Check sheet for the modelled part. Datum: model origin and axes. Units: mm. Face numbers are marked on the shaded views. A direction names the side the tool comes from. Coordinates: 2 decimals unless noted, no trailing zeros. Loops run counter-clockwise (first coordinate to the right, second up) from the corner with the lowest first, then second, coordinate; pieces in that order, holes last. Notation, with made-up numbers: (3.5, 10.25) - (46.5, 10.25) arc R29 ccw to (46.5, 33.25) - close; hole circle Ø2 at (89.25, 16.25). An arc over 180 degrees is marked (long way). Write each question's results on one line, items separated by ' | '. Start each with the question number.
1. Cross-section at C-C (z = -91.5). Record the cut outline in (x, y).
2. Tool access check on the marked faces 1 and 2. Record the directions out of +Z, -Z, +X, -X, +Y, -Y that give a thin tool (end or side, any length) a straight path to the whole face; none if there is none.
3. Thickness scan on line 1 (Y direction, x = -44, z = -1); line 2 (Z direction, x = -59, y = 76.5); line 3 (Y direction, x = -13, z = -303). Record the ranges inside material, lowest first. Write a range as [from, to].
4. Gauge pin test, flat ends, axial feed: P1, Ø8, axis at x = -248, z = -199, coming from the +Y side; P2, Ø7, axis at x = -13.3, y = 179.98, coming from the +Z side; P3, Ø1, axis at y = 183.5, z = -0.5, coming from the -X side. Record the tip position at first contact, or that the pin passes through.
5. Cross-section at B-B (x = -179). Record the cut outline in (y, z).
6. Cross-section at D-D (y = 57). Record the cut outline in (x, z).
7. Cross-section at A-A (y = 98). Record the cut outline in (x, z).
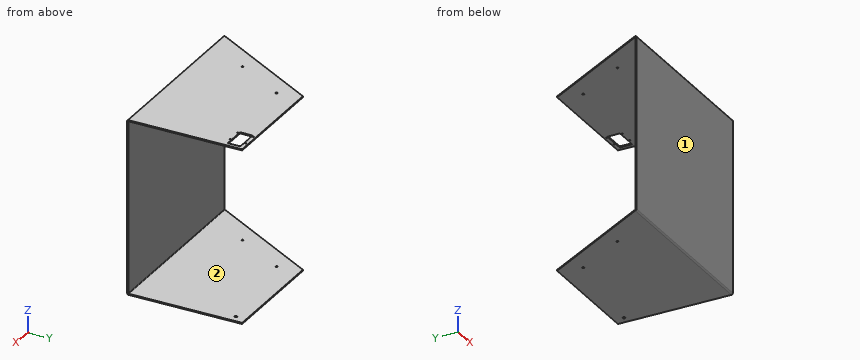
```python
from build123d import *

# Parameters (mm, degrees)
BASE_FLANGE2_DEPTH           = 2
EDGE_FLANGE1_DEPTH           = 309.908043232
EDGE_FLANGE2_STRIP_W         = 9
EDGE_FLANGE2_STRIP_H         = 2
EDGE_FLANGE2_STRIP_CUT_DEPTH = 309.908043232
EDGE_FLANGE2_DEPTH           = 309.908043232
SKETCH23_OUTSIDE_W           = 414.366
SKETCH23_OUTSIDE_H           = 376.458
CUT_EXTRUDE3_DEPTH           = 510.781566222
M3_CLEARANCE_HOLE1_REACH     = 479.133
M3_CLEARANCE_HOLE1_BORE_R    = 1.7
SKETCH50_R                   = 1.2
SKETCH50_W                   = 40
SKETCH50_H                   = 22
CUT_EXTRUDE5_DEPTH           = 10
FILLET1_R                    = 1.5
M4_CLEARANCE_HOLE2_D         = 4.3
M3_CLEARANCE_HOLE2_REACH     = 479.133
M3_CLEARANCE_HOLE2_BORE_R    = 1.7


# Sheet-metal steps are written as plain solids
with BuildPart() as part:
    # Sketch7 → Base-Flange2 (new body)
    with BuildSketch(Plane.XY):
        Polygon((-309.908043232, 0), (-195.602983964, 197.982170213), (0, 197.982170213), (0, 0), align=None)
    extrude(amount=-BASE_FLANGE2_DEPTH)

    # Edge-Flange1 section (across the edge) → Edge-Flange1 (add)
    with BuildSketch(Plane(origin=(0, -0.5, -2), x_dir=(0, 1, 0), z_dir=(-1, 0, 0))):
        with BuildLine():
            Line((-2, 0.5), (-2, 300))
            Line((-2, 300), (0, 300))
            Line((0, 300), (0, 0.5))
            ThreePointArc((0, 0.5), (0.146446609, 0.146446609), (0.5, 0))
            Line((0.5, 0), (0.5, -2))
            ThreePointArc((0.5, -2), (-1.267766953, -1.267766953), (-2, 0.5))
        make_face()
    extrude(amount=EDGE_FLANGE1_DEPTH)

    # Edge-Flange2 strip (across the edge) → Edge-Flange2 strip cut (cut)
    with BuildSketch(Plane(origin=(0, -0.5, -302), x_dir=(0, 0, 1), z_dir=(-1, 0, 0))):
        with Locations((-4, -1)):
            Rectangle(EDGE_FLANGE2_STRIP_W, EDGE_FLANGE2_STRIP_H)
    extrude(amount=EDGE_FLANGE2_STRIP_CUT_DEPTH, mode=Mode.SUBTRACT)

    # Edge-Flange2 section (across the edge) → Edge-Flange2 (add)
    with BuildSketch(Plane(origin=(0, -0.5, -302), x_dir=(0, 0, 1), z_dir=(-1, 0, 0))):
        with BuildLine():
            Line((-2, 0.5), (-2, 270))
            Line((-2, 270), (0, 270))
            Line((0, 270), (0, 0.5))
            ThreePointArc((0, 0.5), (0.146446609, 0.146446609), (0.5, 0))
            Line((0.5, 0), (0.5, -2))
            ThreePointArc((0.5, -2), (-1.267766953, -1.267766953), (-2, 0.5))
        make_face()
    extrude(amount=EDGE_FLANGE2_DEPTH)

    # Sketch23 outside → Cut-Extrude3 (cut, through all)
    with BuildSketch(Plane.XY.offset(-302)):
        with Locations((-154.954, 133.5)):
            Rectangle(SKETCH23_OUTSIDE_W, SKETCH23_OUTSIDE_H)
        Polygon((-309.908043232, 0), (-195.602983964, 197.982170213), (0, 197.982170213), (0, 0), (15.914954138, -38.535343566), (-328.412515317, -22.782185248), align=None, mode=Mode.SUBTRACT)
    extrude(amount=-CUT_EXTRUDE3_DEPTH, mode=Mode.SUBTRACT)

    # M3 Clearance Hole1 bore → M3 Clearance Hole1 (cut, up to next)
    with BuildSketch(Plane(origin=(0, 0, -304), x_dir=(-1, 0, 0), z_dir=(0, 0, -1)), mode=Mode.PRIVATE) as m3_clearance_hole1_sk1:
        with Locations((235.596855298, 71.137815764)):
            Circle(M3_CLEARANCE_HOLE1_BORE_R)
    m3_clearance_hole1_tool1 = extrude(m3_clearance_hole1_sk1.sketch, amount=-M3_CLEARANCE_HOLE1_REACH, mode=Mode.PRIVATE) & part.part
    m3_clearance_hole1 = m3_clearance_hole1_tool1.solids().sort_by_distance((-235.596855, 71.137816, -304))[0]
    add(m3_clearance_hole1, mode=Mode.SUBTRACT)

    # Mirror3: M3 Clearance Hole1 across plane
    add(m3_clearance_hole1.mirror(Plane.XY.offset(-152)), mode=Mode.SUBTRACT)

    # Sketch50 → Cut-Extrude5 (cut)
    with BuildSketch(Plane.XY):
        with Locations((-20, 193.482170213)):
            Circle(SKETCH50_R)
        with Locations((-20, 166.482170213)):
            Circle(SKETCH50_R)
        with Locations((-44, 193.482170213)):
            Circle(SKETCH50_R)
        with Locations((-44, 166.482170213)):
            Circle(SKETCH50_R)
        with Locations((-27, 179.982170213)):
            Rectangle(SKETCH50_W, SKETCH50_H)
    extrude(amount=-CUT_EXTRUDE5_DEPTH, mode=Mode.SUBTRACT)

    # Fillet1
    fillet1_edges = [part.edges().sort_by_distance(p)[0] for p in [
        (-47, 168.982170213, -1),
        (-47, 190.982170213, -1),
        (-7, 190.982170213, -1),
        (-7, 168.982170213, -1),
    ]]
    fillet(fillet1_edges, radius=FILLET1_R)

    # M4 Clearance Hole2 (through all)
    with Locations(Plane(origin=(0, 0, -304), x_dir=(-1, 0, 0), z_dir=(0, 0, -1))):
        with Locations((13.3, 179.982170213)):
            Hole(M4_CLEARANCE_HOLE2_D / 2)

    # M3 Clearance Hole2 bore → M3 Clearance Hole2 (cut, up to next)
    with BuildSketch(Plane(origin=(0, 0, -304), x_dir=(-1, 0, 0), z_dir=(0, 0, -1)), mode=Mode.PRIVATE) as m3_clearance_hole2_sk1:
        with Locations((185.604770825, 157.726646048)):
            Circle(M3_CLEARANCE_HOLE2_BORE_R)
    m3_clearance_hole2_tool1 = extrude(m3_clearance_hole2_sk1.sketch, amount=-M3_CLEARANCE_HOLE2_REACH, mode=Mode.PRIVATE) & part.part
    m3_clearance_hole2 = m3_clearance_hole2_tool1.solids().sort_by_distance((-185.604771, 157.726646, -304))[0]
    add(m3_clearance_hole2, mode=Mode.SUBTRACT)

    # Mirror4: M3 Clearance Hole2 across plane
    add(m3_clearance_hole2.mirror(Plane.XY.offset(-152)), mode=Mode.SUBTRACT)


solid = part.part
```
Established:
1) outline: (-309.91, -2.5) - (0, -2.5) - (0, -0.5) - (-309.91, -0.5) - close
2) face 1: +Z, -Z, +X, -X, -Y | face 2: +X, -X, +Y
3) line 1: [-2, 165.28], [167.68, 168.98], [190.98, 192.28], [194.68, 197.98] | line 2: [-304, -302], [-2, 0] | line 3: [-2, 177.85], [182.11, 197.98]
4) P1: y = -0.5 | P2: z = -302 | P3: x = -204.25
5) outline: (-2.5, -301.5) arc R2.5 ccw to (0, -304) - (197.98, -304) - (197.98, -302) - (0, -302) arc R0.5 cw to (-0.5, -301.5) - (-0.5, -2.5) arc R0.5 cw to (0, -2) - (197.98, -2) - (197.98, 0) - (0, 0) arc R2.5 ccw to (-2.5, -2.5) - close
6) outline: (-277, -304) - (0, -304) - (0, -302) - (-277, -302) - close; (-277, -2) - (0, -2) - (0, 0) - (-277, 0) - close
7) outline: (-253.33, -304) - (0, -304) - (0, -302) - (-253.33, -302) - close; (-253.33, -2) - (0, -2) - (0, 0) - (-253.33, 0) - close
